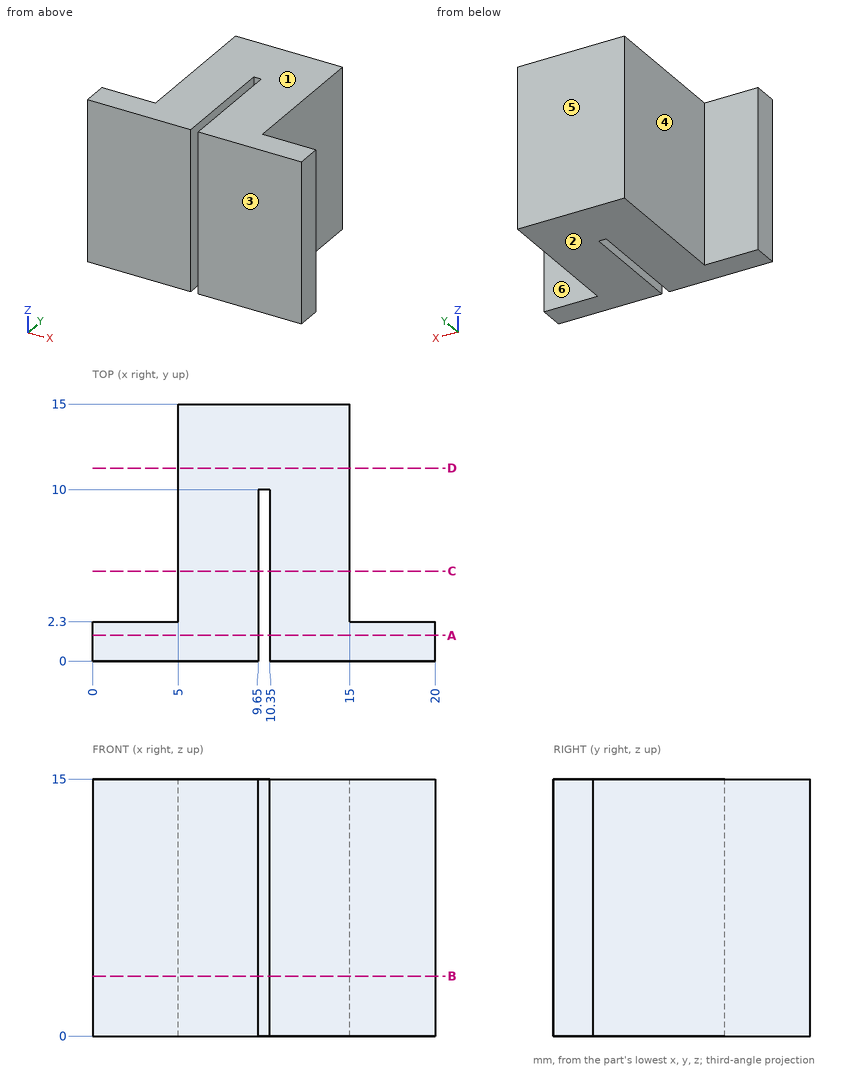
For this review, use the dimensioned drawing (mm, ordinates from the lowest corner) and the shaded views. A direction names the side the tool comes from. Give positions to 0.01 mm unless a question says otherwise; leave off trailing zeros. Order: outer loops, then holes, each group sorted by start corner. A loop starts at its lowest first (then second) coordinate and runs counter-clockwise, first axis right, second up. Notation, with made-up numbers: (38, 48) - (80, 48) arc R5 ccw to (80, 54) - close; hole circle Ø9 at (-29, 34.5). An arc over 180 degrees is marked (long way). Use a Markdown table: item, result. Add a question column.
(1) Add section A-A on y = 1.5. Give the boundary of the cut face in (x, z).
(2) Add section B-B on z = 3.5. Give the boundary of the cut face in (x, y), then the cut area to 3 significant figures.
(3) Wall thickness on probe 1 along X at (y, z) = (5, 5); probe 2 along X at (y, z) = (1, 3.75); probe 3 along Y at (x, z) = (15.25, 8): over which ranges is each line inside the solid? List them lowest first. Write a range as [from, to].
(4) Clearance check with flat-ended pins moving along their axes: P1, Ø4, axis at y = 6, z = 7, coming from the +X side; P2, Ø5, axis at y = 7, z = 5.5, coming from the -X side; P3, Ø1.5, axis at x = 18.5, z = 6, coming from the +Y side. State where each tip first meets the part, or that it passes through.
(5) Add section C-C on y = 5.25. Give the boundary of the cut face in (x, z), then the cut area to 4 significant figures.
(6) Machinability: for the marked faces 4, 5 and 6, which of the approach directions +Z, -Z, +X, -X, +Y, -Y give a long, thin tool a straight path to every point of the face, cutting with its end or side? Answer none if there is none.
(7) Mouldability with a two-part tool opening along Z and no side actions: class the marked faces 1, 2 and 3 as +Z half, -Z half, draft (parallel to the pull), parting line (faces both ways), or undercut.
(8) Add section D-D on y = 11.25. Give the boundary of the cut face in (x, z), then the cut area to 3 significant figures.
Report:
| question | item | result |
|---|---|---|
| 1 | outline | (0, 0) - (9.65, 0) - (9.65, 15) - (0, 15) - close; (10.35, 0) - (20, 0) - (20, 15) - (10.35, 15) - close |
| 2 | outline | (0, 0) - (9.65, 0) - (9.65, 10) - (10.35, 10) - (10.35, 0) - (20, 0) - (20, 2.3) - (15, 2.3) - (15, 15) - (5, 15) - (5, 2.3) - (0, 2.3) - close |
| 2 | area | 166 mm² |
| 3 | probe 1 | x = [5, 9.65], [10.35, 15] |
| 3 | probe 2 | x = [0, 9.65], [10.35, 20] |
| 3 | probe 3 | y = [0, 2.3] |
| 4 | P1 | stops at x = 15 |
| 4 | P2 | stops at x = 5 |
| 4 | P3 | stops at y = 2.3 |
| 5 | outline | (5, 0) - (9.65, 0) - (9.65, 15) - (5, 15) - close; (10.35, 0) - (15, 0) - (15, 15) - (10.35, 15) - close |
| 5 | area | 139.5 mm² |
| 6 | face 4 | +Z, -Z, -X, +Y |
| 6 | face 5 | +Z, -Z, +X, -X, +Y |
| 6 | face 6 | +Z, -Z, +X, +Y |
| 7 | face 1 | +Z half |
| 7 | face 2 | -Z half |
| 7 | face 3 | draft |
| 8 | outline | (5, 0) - (15, 0) - (15, 15) - (5, 15) - close |
| 8 | area | 150 mm² |
